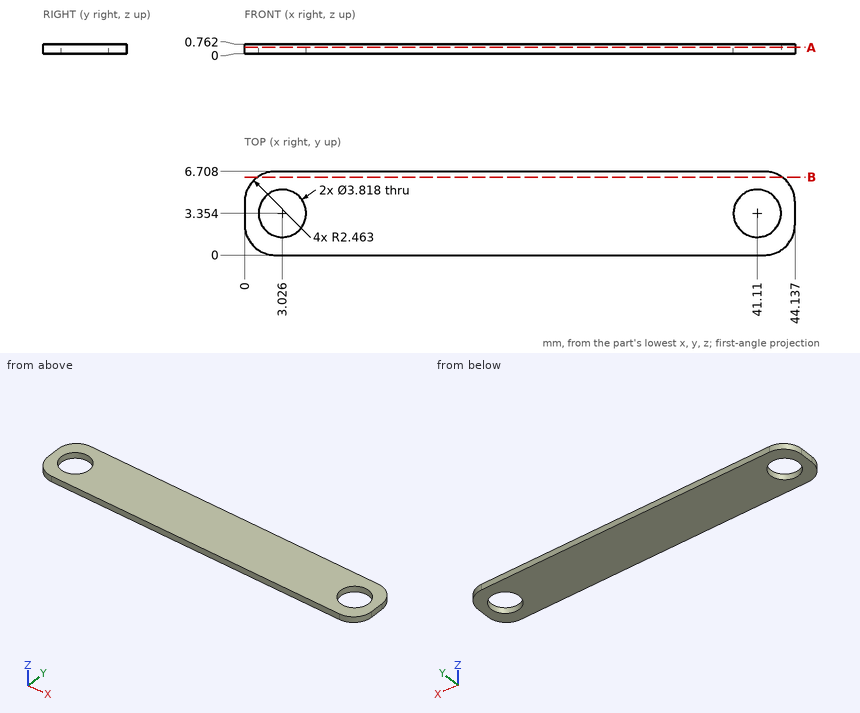
Verification items for this drawing (mm, ordinates from the low corner). Round coordinates to 2 decimals unless told otherwise and drop trailing zeros. Order: outer loops, then holes, each group sorted by start corner. A loop starts at its lowest first (then second) coordinate and runs counter-clockwise, first axis right, second up. Notation, with made-up numbers: M -29.5,55.25 L 3.5,55.25 A32 cw 3.5,93.25 Z; hole C 81.25,35.25 d7. An arc over 180 degrees is marked long. Answer in a Markdown table with one row per item. Add a question column.
Item 1: Material ranges on L1, parallel to X at y = 3.5, z = 0.3 (1 decimal); L2, parallel to X at y = 2.5, z = 0.65 (1 decimal); L3, parallel to X at y = 0.5, z = 0.15 (1 decimal), recorded low to high. Write a range as [from, to].
Item 2: Sectioned sample at A-A, the plane z = 0.5. Enter the section's corners in (x, y) (1 decimal), plus the area to 3 significant figures.
Item 3: Sectioned sample at B-B, the plane y = 6.25. Enter the section's corners in (x, z).
Filled in:
| question | item | result |
|---|---|---|
| 1 | L1 | x = [0, 1.1], [4.9, 39.2], [43, 44.1] |
| 1 | L2 | x = [0, 1.3], [4.7, 39.4], [42.8, 44.1] |
| 1 | L3 | x = [1, 43.2] |
| 2 | outline | M 0,2.5 A2.5 ccw 2.5,0 L 41.7,0 A2.5 ccw 44.1,2.5 L 44.1,4.2 A2.5 ccw 41.7,6.7 L 2.5,6.7 A2.5 ccw 0,4.2 Z; hole C 3,3.4 d3.8; hole C 41.1,3.4 d3.8 |
| 2 | area | 268 mm² |
| 3 | outline | M 1.03,0 L 43.1,0 L 43.1,0.76 L 1.03,0.76 Z |
